```python
from build123d import *

# Parameters (mm, degrees)
BOSS_EXTRUDE1_DEPTH  = 112
SKETCH3_W            = 11
SKETCH3_H            = 11
BOSS_EXTRUDE2_DEPTH  = 4
BOSS_EXTRUDE3_REACH  = 127.251
SKETCH8_W            = 10
SKETCH8_H            = 13
BOSS_EXTRUDE4_DEPTH  = 4
FILLET1_R            = 2
M4_CLEARANCE_HOLE1_D = 4.8
MIRROR1_START        = 13.844633107
MIRROR1_OUTLINE_W    = 4
MIRROR1_OUTLINE_H    = 13
MIRROR1_DEPTH        = 2.782266793
MIRROR1_START_2      = 21.4269001
MIRROR1_2_OUTLINE_W  = 4
MIRROR1_2_OUTLINE_H  = 13
MIRROR1_2_DEPTH      = 0.5999999
MIRROR1_START_3      = 74
MIRROR1_3_DEPTH      = 13
MIRROR1_4_OUTLINE_W  = 4.8000002
MIRROR1_4_OUTLINE_H  = 4
MIRROR1_4_DEPTH      = 4.0999999
MIRROR1_START_4      = 82.9000001
MIRROR1_5_OUTLINE_W  = 4.8000002
MIRROR1_5_OUTLINE_H  = 4
MIRROR1_5_DEPTH      = 4.0999999
MIRROR1_START_5      = 76
MIRROR1_6_OUTLINE_W  = 2
MIRROR1_6_OUTLINE_H  = 4
MIRROR1_6_DEPTH      = 9
MIRROR1_START_6      = -14.0269
MIRROR1_7_DEPTH      = 4
CUT_EXTRUDE2_DEPTH   = 126.72521882
BOSS_EXTRUDE5_START  = -87
BOSS_EXTRUDE5_DEPTH  = 112
SKETCH14_W           = 112
SKETCH14_H           = 14.0269
BOSS_EXTRUDE6_DEPTH  = 1
SKETCH2_R            = 3.025
CUT_EXTRUDE1_DEPTH   = 8
SKETCH15_W           = 10
SKETCH15_H           = 15
SKETCH15_R           = 3.025
BOSS_EXTRUDE7_DEPTH  = 14.0269
SKETCH16_R           = 3.025
CUT_EXTRUDE3_DEPTH   = 8
FILLET2_R            = 2
FILLET3_R            = 1


with BuildPart() as part:
    # Sketch1 → Boss-Extrude1 (new body)
    with BuildSketch(Plane.XY):
        with BuildLine():
            ThreePointArc((0, -14.0269), (-9.918516109, -9.918516109), (-14.0269, 0))
            Line((-14.0269, 0), (-19.0269, 0))
            Line((-19.0269, 0), (-19.0269, -14.0269))
            Line((-19.0269, -14.0269), (0, -14.0269))
        make_face()
        with BuildLine():
            Line((-12.5269, 0), (-14.0269, 0))
            ThreePointArc((-14.0269, 0), (-9.918516109, -9.918516109), (0, -14.0269))
            ThreePointArc((0, -14.0269), (9.918516109, -9.918516109), (14.0269, 0))
            Line((14.0269, 0), (12.5269, 0))
            ThreePointArc((12.5269, 0), (0, -12.5269), (-12.5269, 0))
        make_face()
    extrude(amount=BOSS_EXTRUDE1_DEPTH)

    # Sketch3 → Boss-Extrude2 (add)
    with BuildSketch(Plane.XZ.offset(14.0269)):
        with Locations((-13.5269, 117.5)):
            Rectangle(SKETCH3_W, SKETCH3_H)
    extrude(amount=-BOSS_EXTRUDE2_DEPTH)

    # Sketch7 → Boss-Extrude3 (add, up to next)
    with BuildSketch(Plane.XZ.offset(14.0269), mode=Mode.PRIVATE) as boss_extrude3_sk1:
        Polygon((0, 25), (14.0269, 25), (14.0269, 31.5), (14.0269, 38), (0, 38), align=None)
    boss_extrude3_tool1 = extrude(boss_extrude3_sk1.sketch, amount=-BOSS_EXTRUDE3_REACH, mode=Mode.PRIVATE) - part.part
    add(boss_extrude3_tool1.solids().sort_by_distance((7.01345, -14.0269, 31.5))[0])

    # Sketch8 → Boss-Extrude4 (add)
    with BuildSketch(Plane.XZ.offset(14.0269)):
        with Locations((19.0269, 31.5)):
            Rectangle(SKETCH8_W, SKETCH8_H)
    extrude(amount=-BOSS_EXTRUDE4_DEPTH)

    # Fillet1
    fillet1_edges = [part.edges().sort_by_distance(p)[0] for p in [
        (-19.0269, -12.0269, 123),
        (-8.0269, -12.0269, 123),
        (24.0269, -12.0269, 38),
        (24.0269, -12.0269, 25),
    ]]
    fillet(fillet1_edges, radius=FILLET1_R)

    # M4 Clearance Hole1 (through all)
    with Locations(Plane(origin=(0, -10.0269, 0), x_dir=(1, 0, 0), z_dir=(0, 1, 0))):
        with Locations((-13.5269, -117.5), (19.0269, -31.5)):
            Hole(M4_CLEARANCE_HOLE1_D / 2)



with BuildPart() as body_2:
    # Mirror1: read off the stored shape, not the designer's step
    # Mirror1 outline → Mirror1 (new body)
    with BuildSketch(Plane.YZ.offset(MIRROR1_START)):
        with Locations((-12.0269, 80.5)):
            Rectangle(MIRROR1_OUTLINE_W, MIRROR1_OUTLINE_H)
    extrude(amount=MIRROR1_DEPTH)


with BuildPart() as body_3:
    # Mirror1 2 outline → Mirror1 2 (new body)
    with BuildSketch(Plane.YZ.offset(MIRROR1_START_2)):
        with Locations((-12.0269, 80.5)):
            Rectangle(MIRROR1_2_OUTLINE_W, MIRROR1_2_OUTLINE_H)
    extrude(amount=MIRROR1_2_DEPTH)


with BuildPart() as part_1:
    add(part.part)

    add(body_2.part)  # Mirror1 3 merges body 2
    # Mirror1 3 outline → Mirror1 3 (add)
    with BuildSketch(Plane.XY.offset(MIRROR1_START_3)):
        with BuildLine():
            Line((16.6268999, -10.0269), (14.0269, -10.0269))
            Line((14.0269, -10.0269), (14.0269, 0))
            ThreePointArc((14.0269, 0), (9.918516109, -9.918516109), (0, -14.0269))
            Line((0, -14.0269), (13.844633107, -14.0269))
            Line((13.844633107, -14.0269), (16.6268999, -14.0269))
            Line((16.6268999, -14.0269), (16.6268999, -10.0269))
        make_face()
    extrude(amount=MIRROR1_3_DEPTH)


    add(body_3.part)  # Mirror1 4 merges body 3
    # Mirror1 4 outline → Mirror1 4 (add)
    with BuildSketch(Plane.XY.offset(MIRROR1_START_3)):
        with Locations((19.0269, -12.0269)):
            Rectangle(MIRROR1_4_OUTLINE_W, MIRROR1_4_OUTLINE_H)
    extrude(amount=MIRROR1_4_DEPTH)

    # Mirror1 5 outline → Mirror1 5 (add)
    with BuildSketch(Plane.XY.offset(MIRROR1_START_4)):
        with Locations((19.0269, -12.0269)):
            Rectangle(MIRROR1_5_OUTLINE_W, MIRROR1_5_OUTLINE_H)
    extrude(amount=MIRROR1_5_DEPTH)

    # Mirror1 6 outline → Mirror1 6 (add)
    with BuildSketch(Plane.XY.offset(MIRROR1_START_5)):
        with Locations((23.0269, -12.0269)):
            Rectangle(MIRROR1_6_OUTLINE_W, MIRROR1_6_OUTLINE_H)
    extrude(amount=MIRROR1_6_DEPTH)

    # Mirror1 7 outline → Mirror1 7 (add)
    with BuildSketch(Plane(origin=(0, 0, 0), x_dir=(1, 0, 0), z_dir=(0, 1, 0)).offset(MIRROR1_START_6)):
        with BuildLine():
            ThreePointArc((24.0269, -76), (23.441113562, -74.585786438), (22.0269, -74))
            Line((22.0269, -74), (22.0269, -76))
            Line((22.0269, -76), (24.0269, -76))
        make_face()
        with BuildLine():
            Line((22.0269, -85), (22.0269, -87))
            ThreePointArc((22.0269, -87), (23.441113562, -86.414213562), (24.0269, -85))
            Line((24.0269, -85), (22.0269, -85))
        make_face()
        with BuildLine():
            Line((21.4269001, -82.9000001), (21.4269, -80.5))
            ThreePointArc((21.4269, -80.5), (20.723956275, -82.197056275), (19.0269, -82.9))
            Line((19.0269, -82.9), (21.4269001, -82.9000001))
        make_face()
        with BuildLine():
            ThreePointArc((19.0269, -78.1), (20.723956275, -78.802943725), (21.4269, -80.5))
            Line((21.4269, -80.5), (21.4269001, -78.0999999))
            Line((21.4269001, -78.0999999), (19.0269, -78.1))
        make_face()
        with BuildLine():
            ThreePointArc((16.6269, -80.5), (17.329843725, -78.802943725), (19.0269, -78.1))
            Line((19.0269, -78.1), (16.6268999, -78.0999999))
            Line((16.6268999, -78.0999999), (16.6269, -80.5))
        make_face()
        with BuildLine():
            Line((16.6268999, -82.9000001), (19.0269, -82.9))
            ThreePointArc((19.0269, -82.9), (17.329843725, -82.197056275), (16.6269, -80.5))
            Line((16.6269, -80.5), (16.6268999, -82.9000001))
        make_face()
    extrude(amount=MIRROR1_7_DEPTH)

    # Sketch12 → Cut-Extrude2 (cut, through all)
    with BuildSketch(Plane(origin=(0, -10.0269, 0), x_dir=(1, 0, 0), z_dir=(0, 1, 0))):
        with BuildLine():
            Line((-19.0269, -112), (-19.0269, -121))
            ThreePointArc((-19.0269, -121), (-18.441113562, -122.414213562), (-17.0269, -123))
            Line((-17.0269, -123), (-10.0269, -123))
            ThreePointArc((-10.0269, -123), (-8.612686438, -122.414213562), (-8.0269, -121))
            Line((-8.0269, -121), (-8.0269, -112))
            Line((-8.0269, -112), (-19.0269, -112))
        make_face()
    extrude(amount=-CUT_EXTRUDE2_DEPTH, mode=Mode.SUBTRACT)

    # Sketch13 → Boss-Extrude5 (add)
    with BuildSketch(Plane.XY.offset(87).offset(BOSS_EXTRUDE5_START)):
        with BuildLine():
            Line((14.0269, -14.0269), (14.0269, -10.0269))
            Line((14.0269, -10.0269), (14.0269, 0))
            ThreePointArc((14.0269, 0), (9.918516109, -9.918516109), (0, -14.0269))
            Line((0, -14.0269), (14.0269, -14.0269))
        make_face()
    extrude(amount=BOSS_EXTRUDE5_DEPTH)

    # Sketch14 → Boss-Extrude6 (add)
    with BuildSketch(Plane.ZY.offset(19.0269)):
        with Locations((56, -7.01345)):
            Rectangle(SKETCH14_W, SKETCH14_H)
    extrude(amount=BOSS_EXTRUDE6_DEPTH)

    # Sketch2 → Cut-Extrude1 (cut)
    with BuildSketch(Plane(origin=(0, 0, 0), x_dir=(1, 0, 0), z_dir=(0, 1, 0))):
        with Locations(Location((-16.2769, -25.4, 0), (0, 0, 180))):
            Circle(SKETCH2_R)
        with Locations(Location((-16.2769, -86.6, 0), (0, 0, 180))):
            Circle(SKETCH2_R)
    extrude(amount=-CUT_EXTRUDE1_DEPTH, mode=Mode.SUBTRACT)

    # Sketch15 → Boss-Extrude7 (add)
    # profile 1 of 2: a face of its own
    with BuildSketch(Plane.XZ.offset(14.0269)):
        with Locations((19.0269, 56)):
            Rectangle(SKETCH15_W, SKETCH15_H)
        with Locations((19.0269, 56)):
            Circle(SKETCH15_R, mode=Mode.SUBTRACT)
    # profile 2 of 2: a face of its own
    with BuildSketch(Plane.XZ.offset(14.0269)):
        with Locations((19.0269, 56)):
            Circle(SKETCH15_R)
    extrude(amount=-BOSS_EXTRUDE7_DEPTH)

    # Sketch16 → Cut-Extrude3 (cut)
    with BuildSketch(Plane(origin=(0, 0, 0), x_dir=(1, 0, 0), z_dir=(0, 1, 0))):
        with Locations(Location((19.0269, -56, 0), (0, 0, 270))):
            Circle(SKETCH16_R)
    extrude(amount=-CUT_EXTRUDE3_DEPTH, mode=Mode.SUBTRACT)

    # Fillet2
    fillet2_edges = [part_1.edges().sort_by_distance(p)[0] for p in [
        (24.0269, -7.01345, 63.5),
        (24.0269, -7.01345, 48.5),
        (14.0269, -7.01345, 48.5),
        (14.0269, -7.01345, 63.5),
    ]]
    fillet(fillet2_edges, radius=FILLET2_R)

    # Fillet3
    fillet3_edges = [part_1.edges().sort_by_distance(p)[0] for p in [
        (14.0269, -10.0269, 80.5),
        (14.0269, -12.0269, 25),
        (14.0269, -12.0269, 38),
        (14.0269, -12.0269, 74),
        (14.0269, -12.0269, 87),
        (14.0269, -10.0269, 31.5),
    ]]
    fillet(fillet3_edges, radius=FILLET3_R)


solid = part_1.part
```
The model under review builds one solid part; all positions refer to its coordinate system, in mm. A direction names the side the tool comes from. Round coordinates to 2 decimals unless told otherwise and drop trailing zeros. Loops run counter-clockwise (first coordinate to the right, second up) from the corner with the lowest first, then second, coordinate; pieces in that order, holes last. Notation, with made-up numbers: M 66.5,61 L 72.5,61 A14 ccw 72.5,88 Z; hole C 14,40 d11. An arc over 180 degrees is marked long. Write item = value, one per line.
Item 1: Take a section at C-C on z = 17. Write out the cut boundary in (x, y).
Return value:
outline = M -20.03,-14.03 L 14.03,-14.03 L 14.03,0 L 12.53,0 A12.53 cw -12.53,0 L -20.03,0 Z
Item 2: Insertion check: P1, Ø8, axis at y = -2, z = 29.5, coming from the +X side; P2, Ø1.2, axis at x = 19.5, y = -11.5, coming from the -Z side; P3, Ø5, axis at x = 18, y = -8.5, coming from the +Z side; P4, Ø8, axis at x = 16, y = -9.5, coming from the -Z side. Each pin has a flat end and moves straight along its axis. Give the tip position at first contact, or say it passes through.
Return value:
P1 = 14.03
P2 = 25
P3 = 87
P4 = 0
Item 3: Take a section at A-A on y = -3.5. Write out the cut boundary in (x, z) (3 decimals), then the cut area to 3 significant figures.
Return value:
outline = M -20.027,0 L -12.028,0 L -12.028,112 L -20.027,112 Z; M 12.028,0 L 14.027,0 L 14.027,46.5 A2 cw 16.027,48.5 L 22.027,48.5 A2 ccw 24.027,50.5 L 24.027,61.5 A2 ccw 22.027,63.5 L 16.027,63.5 A2 cw 14.027,65.5 L 14.027,112 L 12.028,112 Z; hole C -16.277,25.4 d6.05; hole C -16.277,86.6 d6.05; hole C 19.027,56 d6.05
area = 1,180 mm2
Item 4: Machinability: for faces 5 (the cylindrical face through (19.16, -3.944, 52.978)), 6 (the cylindrical face through (23.425, -6.915, 49.07)), 7 (the flat face through (18, -12, 25)), 8 (the flat face through (21.5, -10.027, 33)), which of the approach directions +Z, -Z, +X, -X, +Y, -Y give a long, thin tool a straight path to every point of the face, cutting with its end or side? Answer none if there is none.
Return value:
face_5 = +Y
face_6 = +X, +Y, -Y
face_7 = -Z, +X, +Y, -Y
face_8 = -Z, +X, +Y
Item 5: For line 1 (X direction, y = -13.2, z = 31.5); line 2 (X direction, y = -11, z = 32); line 3 (X direction, y = -1, z = 25), list the stretches that pass through material, from the lowest coordinate up. Write a range as [from, to].
Return value:
line_1 = [-20.03, 16.63], [21.43, 24.03]
line_2 = [-20.03, -5.99], [5.99, 16.68], [21.37, 24.03]
line_3 = [-20.03, -19.28], [-13.28, -12.49], [12.49, 14.03]
Item 6: The part is to be moulded in two halves that separate along Z. For faces 1 (the cylindrical face through (23.425, -11.999, 37.43)), 2 (the cylindrical face through (0.275, -12.524, 55.216)), 3 (the flat face through (19, -7, 48.5)), 4 (the cylindrical face through (23.425, -12.055, 86.43)), say which applies: released by +Z, released by -Z, zero draft, split by the parting line, or undercut.
Return value:
face_1 = undercut
face_2 = zero draft
face_3 = undercut
face_4 = released by +Z
Item 7: Take a section at B-B on z = 31.5. Write out the cut boundary in (x, y), then the cut area to 3 significant figures.
Return value:
outline = M -20.03,-14.03 L 16.63,-14.03 L 16.63,-10.03 L 15.03,-10.03 A1 cw 14.03,-9.03 L 14.03,0 L 12.53,0 A12.53 cw -12.53,0 L -20.03,0 Z; M 21.43,-14.03 L 24.03,-14.03 L 24.03,-10.03 L 21.43,-10.03 Z
area = 252 mm2
Item 8: Take a section at D-D on x = 0. Write out the cut boundary in (y, z).
Return value:
outline = M -14.03,0 L -12.53,0 L -12.53,112 L -14.03,112 Z
